Source: three-view drawing plus pictorial views. Frame: mm from the lowest corner of the part. A direction names the side the tool comes from. Round coordinates to 2 decimals unless told otherwise and drop trailing zeros. Loops run counter-clockwise (first coordinate to the right, second up) from the corner with the lowest first, then second, coordinate; pieces in that order, holes last. Notation, with made-up numbers: (43, 13.25) -> (59, 13.25) arc R13 ccw to (59, 22.25) -> close; hole circle Ø3 at (-38, 85.25). An arc over 180 degrees is marked (long way). One line per question, with ' | ' between items. Start each with the question number.
Q1. Access query for the marked faces 5, 6, 7 and 8. Directions: +Z, -Z, +X, -X, +Y, -Y. A direction counts if a zero-diameter tool reaches every point of the face in a straight line with its end or side. Return the directions, or none.
Q2. Cut plane C-C on z = 53.5. Return loops of the section in (x, y), and give its area (3 significant figures).
Q3. Material intervals for L1, parallel to X at y = 133, z = 67.5; L2, parallel to Z at x = 332, y = 48, sorted ascending.
Q4. Cut plane A-A on z = 7. Return loops of the section in (x, y), and give its area (3 significant figures).
Q5. Contact query for flat-ended pins moving along their axis: P1, Ø1, axis at x = 165, y = 53, coming from the +Z side; P2, Ø4, axis at y = 29, z = 29.5, coming from the +X side; P3, Ø20, axis at y = 137.5, z = 57.5, coming from the -X side. Output: stop coordinate, or through.
Q6. Cut plane D-D on x = 247.5. Return loops of the section in (y, z).
Q7. Cut plane B-B on y = 75. Return loops of the section in (x, z).
Q8. Mould query, pull axis Y, two halves, no side actions, for the marked faces 1, 2, 3 and 4. Classes: pulls with the +Y half, pulls with the -Y half, needs draft (parallel to the pull), parting line crosses it, or undercut.
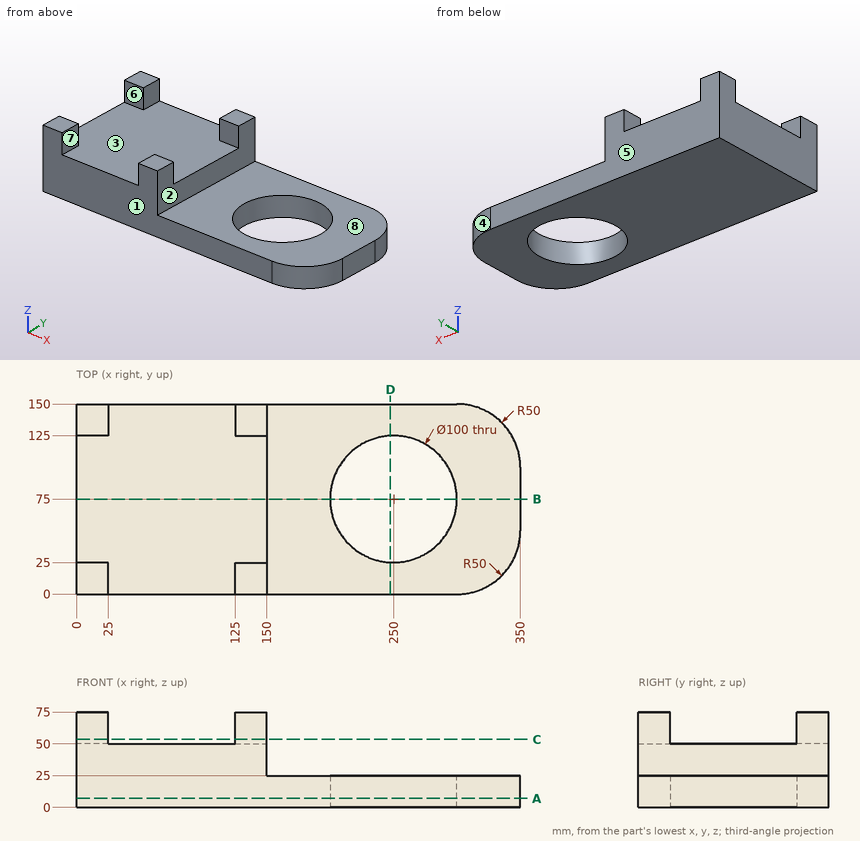
Results:
1) face 5: +Z, -Z, +X, -X, +Y | face 6: +Z, +X, -X | face 7: +Z, +Y, -Y | face 8: +Z, +X, +Y, -Y
2) outline: (0, 0) -> (25, 0) -> (25, 25) -> (0, 25) -> close; (0, 125) -> (25, 125) -> (25, 150) -> (0, 150) -> close; (125, 0) -> (150, 0) -> (150, 25) -> (125, 25) -> close; (125, 125) -> (150, 125) -> (150, 150) -> (125, 150) -> close | area: 2,500 mm^2
3) L1: 0 to 25, 125 to 150 | L2: 0 to 25
4) outline: (0, 0) -> (300, 0) arc R50 ccw to (350, 50) -> (350, 100) arc R50 ccw to (300, 150) -> (0, 150) -> close; hole circle Ø100 at (250, 75) | area: 43,600 mm^2
5) P1: z = 25 | P2: x = 150 | P3: x = 0
6) outline: (0, 0) -> (25.06, 0) -> (25.06, 25) -> (0, 25) -> close; (124.94, 0) -> (150, 0) -> (150, 25) -> (124.94, 25) -> close
7) outline: (0, 0) -> (200, 0) -> (200, 25) -> (150, 25) -> (150, 50) -> (0, 50) -> close; (300, 0) -> (350, 0) -> (350, 25) -> (300, 25) -> close
8) face 1: pulls with the -Y half | face 2: needs draft | face 3: undercut | face 4: pulls with the +Y half
